Verification items for this drawing (mm, ordinates from the low corner). A direction names the side the tool comes from. Give positions to 0.01 mm unless a question says otherwise; leave off trailing zeros. Write each loop counter-clockwise with the first axis right and the second up, starting at its lowest first coordinate (ties: lowest second). Pieces come first, ordered by that corner, then holes. Notation, with made-up numbers: (-9, 13.25) -> (40, 13.25) arc R17 ccw to (40, 22.25) -> close; hole circle Ø6 at (69, 48.25). An arc over 180 degrees is marked (long way). Answer as a JSON object with one key per item and string values.
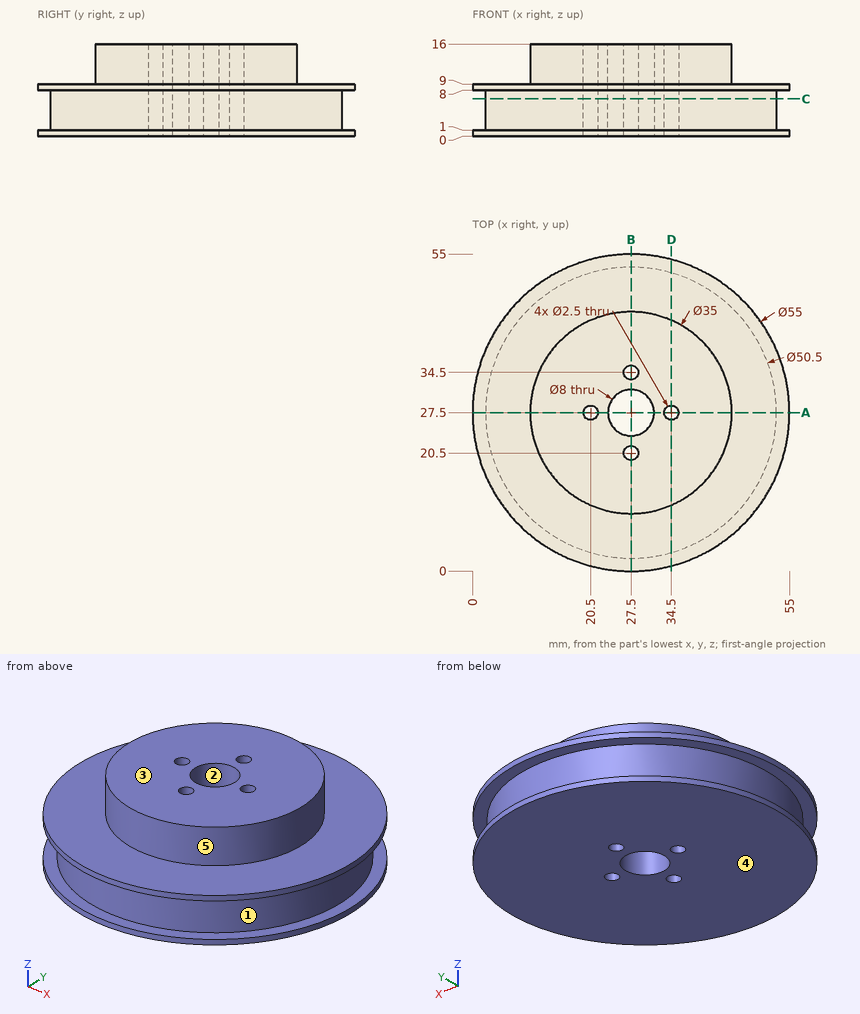
1. Mould release check, pull along Z, two halves, no side actions. Record for the marked faces 1, 2 and 3: released by +Z, released by -Z, zero draft, split by the parting line, or undercut.
Determined:
{"face 1": "undercut", "face 2": "zero draft", "face 3": "released by +Z"}
2. Access from +Z, -Z, +X, -X, +Y, -Y to the whole of each face (thin tool, end or side, straight path). Record for the marked faces 4 and 5.
Determined:
{"face 4": "-Z, +X, -X, +Y, -Y", "face 5": "+Z"}
3. Scan lines: L1, parallel to Y at x = 27.5, z = 5.75; L2, parallel to Y at x = 27.5, z = 11.5; L3, parallel to Z at x = 7, y = 20. Record each from-to range of solid material in increasing order. Write a range as [from, to].
Determined:
{"L1": "[2.25, 19.25], [21.75, 23.5], [31.5, 33.25], [35.75, 52.75]", "L2": "[10, 19.25], [21.75, 23.5], [31.5, 33.25], [35.75, 45]", "L3": "[0, 9]"}
4. Go/stop test with flat-tipped pins: P1, Ø8, axis at y = 45.5, z = 4, coming from the +X side; P2, Ø1, axis at y = 15.5, z = 7, coming from the +X side; P3, Ø12, axis at x = 13.5, y = 9, coming from the -Z side; P4, Ø1, axis at y = 8.5, z = 8, coming from the +X side. Record where each tip stops, or that it passes through.
Determined:
{"P1": "x = 50.31", "P2": "x = 49.98", "P3": "z = 0", "P4": "x = 47.85"}
5. Sectioned sample at C-C, the plane z = 6.5. Enter the section's corners in (x, y), plus the area to 3 significant figures.
Determined:
{"outline": "circle Ø50.5 at (27.5, 27.5); hole circle Ø2.5 at (20.5, 27.5); hole circle Ø8 at (27.5, 27.5); hole circle Ø2.5 at (27.5, 20.5); hole circle Ø2.5 at (27.5, 34.5); hole circle Ø2.5 at (34.5, 27.5)", "area": "1,930 mm^2"}
6. Sectioned sample at A-A, the plane y = 27.5. Enter the section's corners in (x, z).
Determined:
{"outline": "(0, 0) -> (19.25, 0) -> (19.25, 16) -> (10, 16) -> (10, 9) -> (0, 9) -> (0, 8) -> (2.25, 8) -> (2.25, 1) -> (0, 1) -> close; (21.75, 0) -> (23.5, 0) -> (23.5, 16) -> (21.75, 16) -> close; (31.5, 0) -> (33.25, 0) -> (33.25, 16) -> (31.5, 16) -> close; (35.75, 0) -> (55, 0) -> (55, 1) -> (52.75, 1) -> (52.75, 8) -> (55, 8) -> (55, 9) -> (45, 9) -> (45, 16) -> (35.75, 16) -> close"}
7. Sectioned sample at D-D, the plane x = 34.5. Enter the section's corners in (y, z).
Determined:
{"outline": "(0.91, 0) -> (26.25, 0) -> (26.25, 16) -> (11.46, 16) -> (11.46, 9) -> (0.91, 9) -> (0.91, 8) -> (3.24, 8) -> (3.24, 1) -> (0.91, 1) -> close; (28.75, 0) -> (54.09, 0) -> (54.09, 1) -> (51.76, 1) -> (51.76, 8) -> (54.09, 8) -> (54.09, 9) -> (43.54, 9) -> (43.54, 16) -> (28.75, 16) -> close"}
